```python
from build123d import *

# Parameters (mm, degrees)
CYLINDER001_W     = 10
CYLINDER001_H     = 10
CYLINDER001_ANGLE = 320
CYLINDER_R        = 10
CYLINDER_DEPTH    = 10
ARRAY_COUNT       = 8
CYLINDER002_R     = 11
CYLINDER002_DEPTH = 10


with BuildPart() as cilindro:
    # Cylinder001 → Cylinder001 (revolve)
    with BuildSketch(Plane.XZ):
        with Locations((5, 5)):
            Rectangle(CYLINDER001_W, CYLINDER001_H)
    revolve(axis=Axis((0, 0, 0), (0, 0, 1)), revolution_arc=CYLINDER001_ANGLE)


with BuildPart() as array:
    # Cylinder → Cylinder (new body)
    with BuildSketch(Plane.XY):
        Circle(CYLINDER_R)
    extrude(amount=CYLINDER_DEPTH)

    # Cut: cut Cilindro
    add(cilindro.part, mode=Mode.SUBTRACT)


with BuildPart() as array_1:
    # Cut placement: moved
    add(array.part.moved(Location((0, 0, 3))))

    # Array: Array ×8 about axis
    array_axis = Axis((0, 0, 0), (0, 0, 1))


with BuildPart() as array_2:
    add(array_1.part)
    for i in range(1, ARRAY_COUNT):
        add(array_1.part.rotate(array_axis, i * 360 / ARRAY_COUNT))


with BuildPart() as cut001:
    # Cylinder002 → Cylinder002 (new body)
    with BuildSketch(Plane.XY):
        Circle(CYLINDER002_R)
    extrude(amount=CYLINDER002_DEPTH)

    # Cut001: cut Array
    add(array_2.part, mode=Mode.SUBTRACT)


solid = cut001.part
```
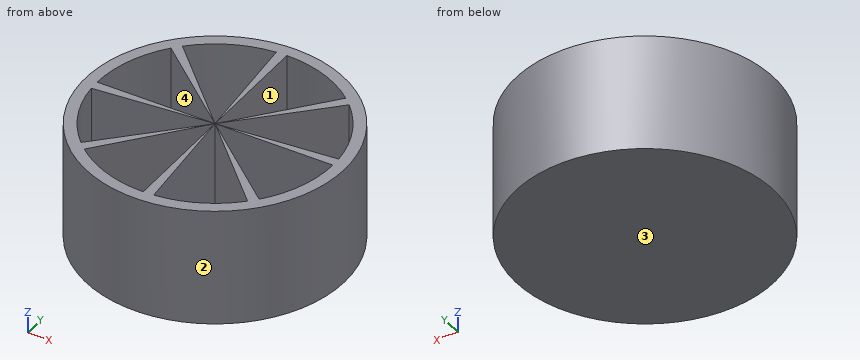
Here's how the part is built. I have some questions about the finished solid (model axes, mm). Face numbers are marked on the shaded views. Round coordinates to 2 decimals unless told otherwise and drop trailing zeros. Write each loop counter-clockwise with the first axis right and the second up, starting at its lowest first coordinate (ties: lowest second). Pieces come first, ordered by that corner, then holes.
Q1. Will these pins go through, and if not, where does the flat tip stop? P1, Ø1.5, axis at y = 5.5, z = 6, coming from the -X side; P2, Ø1, axis at y = -7, z = 1.5, coming from the +X side; P3, Ø1.5, axis at x = 3.5, z = 5.5, coming from the -Y side.
Q2. If we section it at B-B on y = 3.5: Write out the boundary of the cut face in (x, z).
Q3. If we section it at D-D on y = -2.25: Write out the boundary of the cut face in (x, z).
Q4. If we mould it in two halves opening along X, with no side actions, what happens to the marked faces 1, 2, 3 and 4? For each: +X half, -X half, draft (parallel to the pull), parting line (faces both ways), or undercut.
Q5. If we section it at C-C on x = 9: Write out the boundary of the cut face in (y, z).
Q6. Please list where these lines run through material, in increasing order: probe 1 along X at (y, z) = (8, 5); probe 2 along X at (y, z) = (4.75, 6.75); probe 3 along X at (y, z) = (-8.5, 5.5).
Answer below:
1. P1: stops at x = -9.92
1. P2: stops at x = 8.87
1. P3: stops at y = -10.65
2. outline: (-10.43, 0) - (10.43, 0) - (10.43, 10) - (9.37, 10) - (9.37, 3) - (3.5, 3) - (3.5, 10) - (2.94, 10) - (2.94, 3) - (0, 3) - (0, 10) - (-0.31, 10) - (-0.31, 3) - (-3.5, 3) - (-3.5, 10) - (-4.17, 10) - (-4.17, 3) - (-9.37, 3) - (-9.37, 10) - (-10.43, 10) - close
3. outline: (-10.77, 0) - (10.77, 0) - (10.77, 10) - (9.74, 10) - (9.74, 3) - (2.68, 3) - (2.68, 10) - (2.25, 10) - (2.25, 3) - (0.2, 3) - (0.2, 10) - (0, 10) - (0, 3) - (-1.89, 3) - (-1.89, 10) - (-2.25, 10) - (-2.25, 3) - (-9.74, 3) - (-9.74, 10) - (-10.77, 10) - close
4. face 1: undercut
4. face 2: parting line
4. face 3: draft
4. face 4: undercut
5. outline: (-6.32, 0) - (6.32, 0) - (6.32, 10) - (4.36, 10) - (4.36, 3) - (0.79, 3) - (0.79, 10) - (0, 10) - (0, 3) - (-4.36, 3) - (-4.36, 10) - (-6.32, 10) - close
6. probe 1: x = -7.55 to -6, -0.7 to 0, 6 to 7.55
6. probe 2: x = -9.92 to -8.8, -5.66 to -4.75, -0.42 to 0, 3.99 to 4.75, 8.8 to 9.92
6. probe 3: x = -6.98 to -5.27, 0 to 0.74, 5.27 to 6.98
